Geometry check sheet. Reference: the model listing, model coordinates, mm. Face numbers are marked on the shaded views. A direction names the side the tool comes from. Round coordinates to 2 decimals unless told otherwise and drop trailing zeros. Write each loop counter-clockwise with the first axis right and the second up, starting at its lowest first coordinate (ties: lowest second). Pieces come first, ordered by that corner, then holes. Notation, with made-up numbers: (67.25, 48) - (89.25, 48) arc R9 ccw to (89.25, 65) - close; hole circle Ø6 at (51.25, 24.25). An arc over 180 degrees is marked (long way). Return JSON: item names as keys, results as strings. Group by question number.
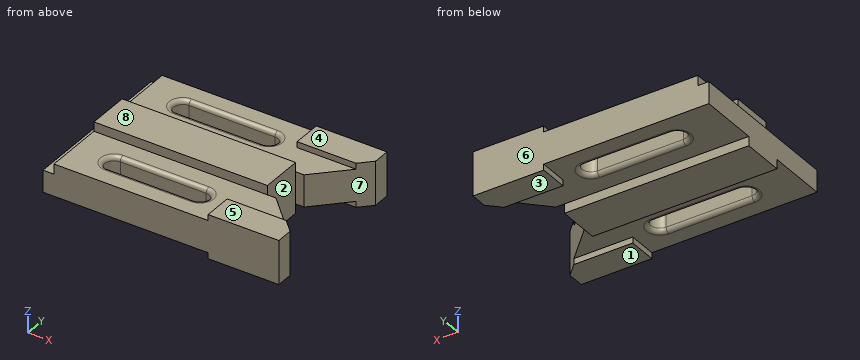
from build123d import *

# Parameters (mm, degrees)
SKETCH1_W           = 109.5
SKETCH1_H           = 12.5
BOSS_EXTRUDE1_DEPTH = 15
BOSS_EXTRUDE2_DEPTH = 9.5
BOSS_EXTRUDE3_DEPTH = 13
SKETCH2_W           = 6.5
SKETCH2_H           = 11.5
CUT_EXTRUDE1_DEPTH  = 149.758193052
FILLET1_R           = 2.5


with BuildPart() as part:
    # Sketch1 → Boss-Extrude1 (new, symmetric)
    with BuildSketch(Plane.XY):
        with Locations((54.75, 6.25)):
            Rectangle(SKETCH1_W, SKETCH1_H)
    extrude(amount=BOSS_EXTRUDE1_DEPTH, both=True)

    # Sketch1<3> → Boss-Extrude2 (add, symmetric)
    with BuildSketch(Plane.XY):
        Polygon((0, 12.5), (109.5, 12.5), (114.5, 12.5), (133, 31), (98, 31), (98, 48), (0, 48), align=None)
        with BuildLine():
            ThreePointArc((30.5, 25), (25, 30.5), (30.5, 36))
            Line((30.5, 36), (81.5, 36))
            ThreePointArc((81.5, 36), (87, 30.5), (81.5, 25))
            Line((81.5, 25), (30.5, 25))
        make_face(mode=Mode.SUBTRACT)
    extrude(amount=BOSS_EXTRUDE2_DEPTH, both=True)

    # Sketch1<4> → Boss-Extrude3 (add, symmetric)
    with BuildSketch(Plane.XY):
        Polygon((98, 31), (133, 31), (140, 38), (140, 48), (98, 48), align=None)
    extrude(amount=BOSS_EXTRUDE3_DEPTH, both=True)

    # Sketch2 → Cut-Extrude1 (cut, through all)
    with BuildSketch(Plane(origin=(0, 48, 0), x_dir=(1, 0, 0), z_dir=(0, 1, 0))):
        with Locations((3.25, -9.25)):
            Rectangle(SKETCH2_W, SKETCH2_H)
    extrude(amount=-CUT_EXTRUDE1_DEPTH, mode=Mode.SUBTRACT)

    # Fillet1
    fillet1_edges = [part.edges().sort_by_distance(p)[0] for p in [
        (87, 30.5, 9.5),
        (56, 25, 9.5),
        (25, 30.5, 9.5),
        (56, 36, -9.5),
        (56, 36, 9.5),
        (87, 30.5, -9.5),
        (25, 30.5, -9.5),
        (56, 25, -9.5),
    ]]
    fillet(fillet1_edges, radius=FILLET1_R)

    # Mirror2: part across plane


with BuildPart() as part_1:
    add(part.part)
    add(part.part.mirror(Plane(origin=(0, 0, 15), x_dir=(0, 0, 1), z_dir=(0, -1, 0))))


solid = part_1.part
1. Mould release check, pull along Y, two halves, no side actions. Record for the marked faces 6, 7 and 8: pulls with the +Y half, pulls with the -Y half, needs draft (parallel to the pull), parting line crosses it, or undercut.
2. Section check D-D (y = -9.5). Enter the section's corners in (x, z).
3. Depth check by flat-ended pin: pin 1 Ø10 at (x, y) = (37.5, -24) entering from -Z; pin 2 Ø5 at (y, z) = (22.5, -5) entering from +X; pin 3 Ø18 at (x, y) = (89, -22.5) entering from +Z. Enter the tip coordinate at first touch or a pass-through.
4. Section check C-C (y = 19). Enter the section's corners in (x, z).
5. Tool access check on the marked faces 1, 2, 3, 4 and 5. Record the directions out of +Z, -Z, +X, -X, +Y, -Y that give a thin tool (end or side, any length) a straight path to the whole face; none if there is none.
6. Material ranges on line 1 along Y through (x, z) = (123, 11.75); line 2 along Y through (x, z) = (69.5, 8.5); line 3 along Z through (x, y) = (25.5, -43.5), recorded low to high.
7. Section check B-B (x = 13). Enter the section's corners in (y, z), and give its area (3 significant figures).
8. Section check A-A (x = 52). Enter the section's corners in (y, z).
Result sheet:
{
 "1": {"face 6": "pulls with the +Y half", "face 7": "undercut", "face 8": "needs draft"},
 "2": {"outline": "(0, -15) - (109.5, -15) - (109.5, 15) - (6.5, 15) - (6.5, 3.5) - (0, 3.5) - close"},
 "3": {"pin 1": "stops at z = -9.5", "pin 2": "stops at x = 127", "pin 3": "stops at z = 9.5"},
 "4": {"outline": "(0, -9.5) - (121, -9.5) - (121, 9.5) - (6.5, 9.5) - (6.5, 3.5) - (0, 3.5) - close"},
 "5": {"face 1": "-Z, +X, -X, -Y", "face 2": "+Z, -Z, +X", "face 3": "-Z, +X, -X, +Y", "face 4": "+Z, +X, -X, +Y", "face 5": "+Z, +X, -X, -Y"},
 "6": {"line 1": "y = -48 to -31, 31 to 48", "line 2": "y = -48 to -36.5, -24.5 to 24.5, 36.5 to 48", "line 3": "z = -9.5 to 9.5"},
 "7": {"outline": "(-48, -9.5) - (-12.5, -9.5) - (-12.5, -15) - (12.5, -15) - (12.5, -9.5) - (48, -9.5) - (48, 9.5) - (12.5, 9.5) - (12.5, 15) - (-12.5, 15) - (-12.5, 9.5) - (-48, 9.5) - close", "area": "2,100 mm²"},
 "8": {"outline": "(-48, -9.5) - (-38.5, -9.5) arc R2.5 ccw to (-36, -7) - (-36, 7) arc R2.5 ccw to (-38.5, 9.5) - (-48, 9.5) - close; (-25, -7) arc R2.5 ccw to (-22.5, -9.5) - (-12.5, -9.5) - (-12.5, -15) - (12.5, -15) - (12.5, -9.5) - (22.5, -9.5) arc R2.5 ccw to (25, -7) - (25, 7) arc R2.5 ccw to (22.5, 9.5) - (12.5, 9.5) - (12.5, 15) - (-12.5, 15) - (-12.5, 9.5) - (-22.5, 9.5) arc R2.5 ccw to (-25, 7) - close; (36, -7) arc R2.5 ccw to (38.5, -9.5) - (48, -9.5) - (48, 9.5) - (38.5, 9.5) arc R2.5 ccw to (36, 7) - close"}
}
